Autodesk Inventor part; units mm, degrees
ref_plane "YZ Plane" through (0, 0, 0) normal (1, 0, 0) x (0, 1, 0)
ref_plane "XZ Plane" through (0, 0, 0) normal (0, 1, 0) x (-1, 0, 0)
ref_plane "XY Plane" through (0, 0, 0) normal (0, 0, 1) x (1, 0, 0)
sketch "スケッチ1" plane through (0, 0, 0) normal (0, 0, 1) x (1, 0, 0)
  circle A0 centre (10.6603, 9.9994) radius 2.15
  circle A1 centre (179.6946, 9.9994) radius 2.15
  circle A2 centre (100.6774, 40.6494) radius 2.15
  circle A3 centre (80.1774, 38.4994) radius 2.15
  circle A4 centre (50.1774, 38.4994) radius 2.15
  circle A5 centre (19.0782, 4.9994) radius 2.15
  circle A6 centre (171.2766, 4.9994) radius 2.15
  circle A7 centre (171.0615, 37.0055) radius 2.15
  circle A8 centre (5.8155, 23.9994) radius 2.15
  circle A9 centre (5.8155, 37.9994) radius 2.15
  circle A10 centre (184.5394, 23.9994) radius 2.15
  circle A11 centre (184.5394, 37.9994) radius 2.15
  circle A12 centre (155.1774, 19.9994) radius 5
  circle A13 centre (95.1774, 19.9994) radius 9.5
  circle A14 centre (65.1774, 19.9994) radius 9.5
  circle A15 centre (35.1774, 19.9994) radius 5
  circle A16 centre (132.9274, 13.826) radius 1.6
  circle A17 centre (109.6774, 27.2494) radius 1.6
  line L0 (105.6774, 48.2494) -> (144.6774, 48.2494)
  line L1 (144.6774, 48.2494) -> (144.6774, 27.2494)
  arc A18 (105.6774, 27.2494) -> (144.6774, 27.2494) centre (125.1774, 27.2494) ccw
  line L2 (105.6774, 27.2494) -> (105.6774, 48.2494)
  circle A19 centre (125.1774, 19.9994) radius 6.5
  line L3 (0, 44.9994) -> (0, 14.9994)
  line L4 (0, 14.9994) -> (5.6908, 10.5508)
  arc A20 (5.6908, 10.5508) -> (13.7466, 6.0657) centre (10.6603, 9.9994) ccw
  line L5 (13.7466, 6.0657) -> (14.154, 5.8665)
  arc A21 (14.154, 5.8665) -> (24.0782, 4.9994) centre (19.0782, 4.9994) ccw
  line L6 (190.3548, 44.9994) -> (190.3548, 14.9994)
  line L7 (190.3548, 14.9994) -> (184.6641, 10.5508)
  arc A22 (176.6082, 6.0657) -> (184.6641, 10.5508) centre (179.6946, 9.9994) ccw
  line L8 (176.6082, 6.0657) -> (176.2009, 5.8665)
  arc A23 (166.2766, 4.9994) -> (176.2009, 5.8665) centre (171.2766, 4.9994) ccw
  line L9 (24.0782, 4.9994) -> (166.2766, 4.9994)
  line L10 (0, 44.9994) -> (190.3548, 44.9994)
  line L11 (0, 44.9994) -> (190.3548, 44.9994)
  line L12 (190.3548, 44.9994) -> (190.3548, 14.9994)
  line L13 (0, 44.9994) -> (0, 14.9994)
  line L14 (5.6908, 10.5508) -> (0, 14.9994)
  line L15 (24.0782, 4.9994) -> (166.2766, 4.9994)
  line L16 (184.6641, 10.5508) -> (190.3548, 14.9994)
  arc A24 (8.228, 5.6308) -> (13.7466, 6.0657) centre (10.6603, 9.9994) ccw
  line L17 (13.7466, 6.0657) -> (14.154, 5.8665)
  arc A25 (166.2766, 4.9994) -> (176.2009, 5.8665) centre (171.2766, 4.9994) ccw
  arc A26 (176.6082, 6.0657) -> (184.6641, 10.5508) centre (179.6946, 9.9994) ccw
  line L18 (176.6082, 6.0657) -> (176.2009, 5.8665)
  arc A27 (16.5868, 0.6644) -> (24.0782, 4.9994) centre (19.0782, 4.9994) ccw
  circle A28 centre (5.8155, 37.9994) radius 2.15
  circle A29 centre (5.8155, 23.9994) radius 2.15
  circle A30 centre (10.6603, 9.9994) radius 2.15
  circle A31 centre (19.0782, 4.9994) radius 2.15
  circle A32 centre (50.1774, 38.4994) radius 2.15
  circle A33 centre (80.1774, 38.4994) radius 2.15
  circle A34 centre (100.6774, 40.6494) radius 2.15
  circle A35 centre (171.0615, 37.0055) radius 2.15
  circle A36 centre (184.5394, 37.9994) radius 2.15
  circle A37 centre (184.5394, 23.9994) radius 2.15
  circle A38 centre (179.6946, 9.9994) radius 2.15
  circle A39 centre (171.2766, 4.9994) radius 2.15
  circle A40 centre (109.6774, 27.2494) radius 1.6
  circle A41 centre (132.9274, 13.826) radius 1.6
  circle A42 centre (125.1774, 19.9994) radius 6.5
  point P0 (0, 0)
  dimension "d0" = 10
  dimension "d1" = 19
sketch "スケッチ2" plane through (0, 0, 0) normal (0, 0, 1) x (1, 0, 0)
  point P0 (0, 0)
extrude "押し出し1" add sketch "スケッチ1" along normal blind 5.5 contours L10 L1 A18 L2 | L2 A18 L1 L10 L6 L7 A22 L8 A23 L9 A21 L5 A20 L4 L3
properties part number "1枚目" material "MDF 中密度繊維ボード"
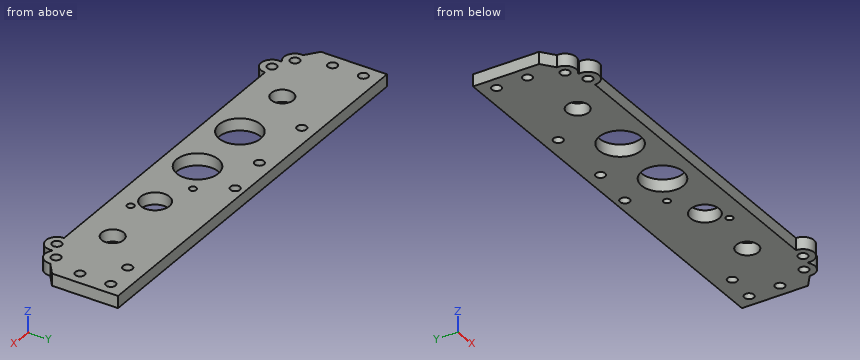
Verification items for the finished model (mm, model axes). Round coordinates to 2 decimals unless told otherwise and drop trailing zeros. Order: outer loops, then holes, each group sorted by start corner. A loop starts at its lowest first (then second) coordinate and runs counter-clockwise, first axis right, second up.
1. Section check B-B on z = 2.25. State how many separate pieces and enclosed holes the cut face has, then the cut area to 3 significant figures.
Final values:
separate pieces: 1
enclosed holes: 19
area: 6,540 mm2
2. Section check C-C on x = 36.5. Record the cut outline in (y, z).
Final values:
outline: (5, 0) - (15.18, 0) - (15.18, 5.5) - (5, 5.5) - close; (24.82, 0) - (45, 0) - (45, 5.5) - (24.82, 5.5) - close
3. Thickness scan on L1, parallel to X at y = 20.5, z = 4.75; L2, parallel to Y at x = 100, z = 4.1; L3, parallel to X at y = 16, z = 3.6. Record the ranges inside material, lowest first.
Final values:
L1: x = 0 to 30.2, 40.15 to 55.69, 74.66 to 85.69, 104.66 to 118.7, 131.66 to 150.2, 160.15 to 190.35
L2: y = 5 to 11.81, 28.18 to 38.61, 42.69 to 45
L3: x = 0 to 32.18, 38.18 to 56.56, 73.79 to 86.56, 103.79 to 120.05, 130.3 to 152.18, 158.18 to 190.35
4. Go/stop test with flat-tipped pins: P1, Ø9, axis at x = 155.18, y = 20, coming from the -Z side; P2, Ø2, axis at x = 145, z = 3, coming from the -Y side. Record where each tip stops, or that it passes through.
Final values:
P1: passes through
P2: stops at y = 5
5. Section check A-A on x = 122. Record the cut outline in (y, z), then the cut area to 3 significant figures.
Final values:
outline: (5, 0) - (14.33, 0) - (14.33, 5.5) - (5, 5.5) - close; (25.67, 0) - (45, 0) - (45, 5.5) - (25.67, 5.5) - close
area: 158 mm2
